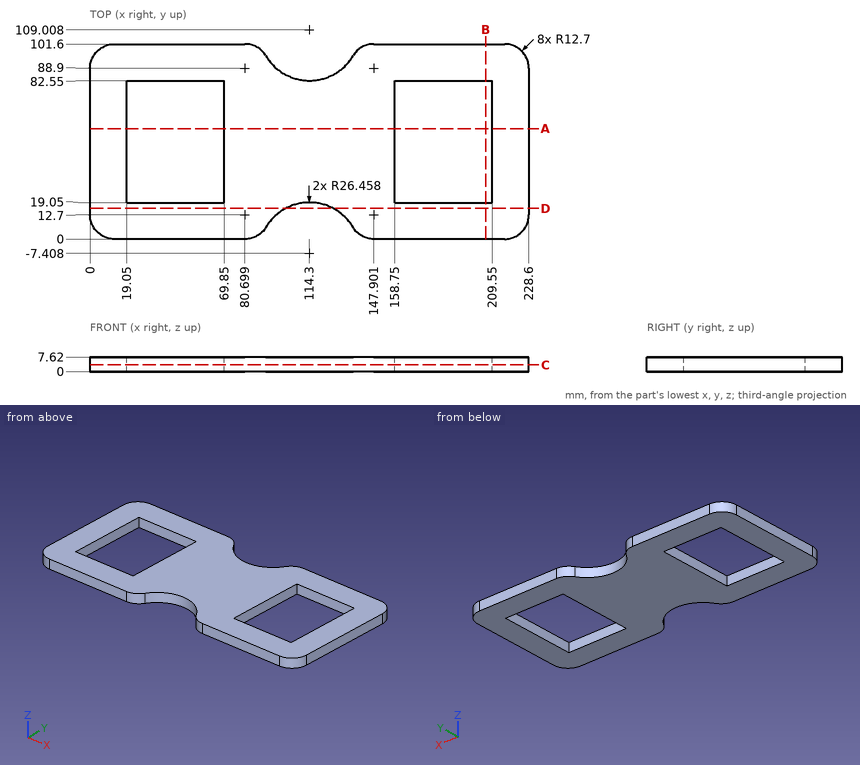
The drawing under review shows one solid part. Ordinate dimensions are in mm from its lowest x, y, z. Coordinates: 2 decimals unless noted, no trailing zeros. Order: outer loops, then holes, each group sorted by start corner. A loop starts at its lowest first (then second) coordinate and runs counter-clockwise, first axis right, second up. Notation, with made-up numbers: (79.5, 6) -> (117.5, 6) arc R21 cw to (117.5, 21) -> close; hole circle Ø7 at (-27.75, -38). An arc over 180 degrees is marked (long way). One line per item, written item: value.
1) We need section A-A, the plane y = 57.5. Give the boundary of the cut face in (x, z), then the cut area to 3 significant figures.
Output values:
outline: (0, 0) -> (19.05, 0) -> (19.05, 7.62) -> (0, 7.62) -> close; (69.85, 0) -> (158.75, 0) -> (158.75, 7.62) -> (69.85, 7.62) -> close; (209.55, 0) -> (228.6, 0) -> (228.6, 7.62) -> (209.55, 7.62) -> close
area: 968 mm2
2) Clearance check with a flat-ended pin moving along its axis: P1, Ø2, axis at y = 11, z = 5, coming from the -X side. State where the tip first meets the part, or that it passes through.
Output values:
P1: stops at x = 0.02
3) We need section D-D, the plane y = 16. Give the boundary of the cut face in (x, z), then the cut area to 3 significant figures.
Output values:
outline: (0, 0) -> (101.97, 0) -> (101.97, 7.62) -> (0, 7.62) -> close; (126.63, 0) -> (228.6, 0) -> (228.6, 7.62) -> (126.63, 7.62) -> close
area: 1,550 mm2
4) We need section C-C, the plane z = 3.5. Give the boundary of the cut face in (x, y), then the cut area to 3 significant figures.
Output values:
outline: (0, 12.7) arc R12.7 ccw to (12.7, 0) -> (80.7, 0) arc R12.7 ccw to (91.6, 6.18) arc R26.46 cw to (137, 6.18) arc R12.7 ccw to (147.9, 0) -> (215.9, 0) arc R12.7 ccw to (228.6, 12.7) -> (228.6, 88.9) arc R12.7 ccw to (215.9, 101.6) -> (147.9, 101.6) arc R12.7 ccw to (137, 95.42) arc R26.46 cw to (91.6, 95.42) arc R12.7 ccw to (80.7, 101.6) -> (12.7, 101.6) arc R12.7 ccw to (0, 88.9) -> close; hole (19.05, 19.05) -> (69.85, 19.05) -> (69.85, 82.55) -> (19.05, 82.55) -> close; hole (158.75, 19.05) -> (209.55, 19.05) -> (209.55, 82.55) -> (158.75, 82.55) -> close
area: 15,200 mm2
5) To check wall thickness, follow probe 1 along X at (y, z) = (77, 4.5); probe 2 along Y at (x, z) = (41, 2.5); probe 3 along Y at (x, z) = (216, 6.5). State the ranges of each line that lie inside material, in increasing order. Write a range as [from, to].
Output values:
probe 1: x = [0, 19.05], [69.85, 158.75], [209.55, 228.6]
probe 2: y = [0, 19.05], [82.55, 101.6]
probe 3: y = [0, 101.6]
6) We need section B-B, the plane x = 206. Give the boundary of the cut face in (y, z).
Output values:
outline: (0, 0) -> (19.05, 0) -> (19.05, 7.62) -> (0, 7.62) -> close; (82.55, 0) -> (101.6, 0) -> (101.6, 7.62) -> (82.55, 7.62) -> close
